Input: part model. Units: mm. Frame: model coordinates. A direction names the side the tool comes from. Give positions to 0.01 mm unless a question says otherwise; leave off trailing zeros. Loops run counter-clockwise (first coordinate to the right, second up) from the corner with the lowest first, then second, coordinate; pieces in that order, holes last. Notation, with made-up numbers: M 78,-28 L 82,-28 A21 cw 82,3 Z; hole C -21.5,55.25 d8. An arc over 180 degrees is marked long. One line per item, written item: value. Start each with the question number.
(1) Pin query (flat end, axial travel): P1, Ø4, axis at y = 87, z = -4, coming from the -X side; P2, Ø4, axis at y = 87.5, z = -4, coming from the -X side; P3, Ø3, axis at x = -11, z = -5, coming from the -Y side; P4, Ø10, axis at x = 0.5, y = 96, coming from the +Z side. Return the tip coordinate at first contact, or that it passes through.
(2) Section C-C on x = -9. Output: boundary loops of the cut face in (y, z).
(3) Section A-A on y = 94.5. Output: boundary loops of the cut face in (x, z).
(4) Pull-direction query (Y, two-part tool) for faces 1 (the flat face through (-9, 98.264, -5)), 2 (the cylindrical face through (-14.457, 98.836, -4.93)), 3 (the flat face through (2.38, 84.51, -4.93)); classes: released by +Y, released by -Y, zero draft, split by the parting line, or undercut.
(5) Section B-B on y = 92.25. Output: boundary loops of the cut face in (x, z), plus the area to 4 significant figures.
(6) Ray query, line 1 along X through (y, z) = (96.5, -1.25); line 2 along X through (y, z) = (85.5, -3.25); line 3 along Y through (x, z) = (-1, -6.75). Return the intervals inside material, ascending. Write a range as from..to.
(7) Access query for faces 4 (the flat face through (1.397, 86.815, -4.93)), 5 (the flat face through (-1.073, 83, -5)), 6 (the flat face through (-13.42, 87.23, -4.93)). Directions: +Z, -Z, +X, -X, +Y, -Y. A direction counts if a zero-diameter tool reaches every point of the face in a straight line with its end or side. Return the directions, or none.
```python
from build123d import *

# Parameters (mm, degrees)
BOSS_EXTRUDE1_DEPTH = 10


# Read off the part's stored shape, not the designer's step: Imported1
with BuildPart() as part:
    # Sketch5 → Boss-Extrude1 (new body)
    with BuildSketch(Plane.XY):
        with BuildLine():
            Line((-6.05700016, 98.805000305), (-6.127999783, 98.944999695))
            Line((-6.127999783, 98.944999695), (-6.152999878, 99.099998474))
            Line((-6.152999878, 99.099998474), (-6.127999783, 99.255996704))
            Line((-6.127999783, 99.255996704), (-6.123951545, 99.263979588))
            Line((-6.123951545, 99.263979588), (-13.408000231, 99.263979588))
            ThreePointArc((-13.408000231, 99.263979588), (-14.468660403, 98.82463976), (-14.908000231, 97.763979588))
            Line((-14.908000231, 97.763979588), (-14.908000231, 93.983181661))
            ThreePointArc((-14.908000231, 93.983181661), (-14.890789829, 93.756609361), (-14.839553555, 93.535236262))
            Line((-14.839553555, 93.535236262), (-13.37100029, 88.842002869))
            Line((-13.37100029, 88.842002869), (-13.322039604, 88.843772888))
            Line((-13.322039604, 88.843772888), (-13.524080276, 85.57485199))
            Line((-13.524080276, 85.57485199), (-13.550000191, 84.919998169))
            Line((-13.550000191, 84.919998169), (-13.409000397, 84.103996277))
            Line((-13.409000397, 84.103996277), (-12.994999886, 83.488998413))
            Line((-12.994999886, 83.488998413), (-12.32199955, 83.050003052))
            Line((-12.32199955, 83.050003052), (-11.402999878, 82.754997253))
            Line((-11.402999878, 82.754997253), (-10.253000259, 82.577003479))
            Line((-10.253000259, 82.577003479), (-10.078000069, 82.565231323))
            Line((-10.078000069, 82.565231323), (-10.078000069, 83.426826477))
            Line((-10.078000069, 83.426826477), (-10.673000336, 83.518997192))
            Line((-10.673000336, 83.518997192), (-11.477000237, 83.777000427))
            Line((-11.477000237, 83.777000427), (-12.065999985, 84.162002563))
            Line((-12.065999985, 84.162002563), (-12.428999901, 84.699996948))
            Line((-12.428999901, 84.699996948), (-12.552000046, 85.414001465))
            Line((-12.552000046, 85.414001465), (-12.44299984, 88.178001404))
            Line((-12.44299984, 88.178001404), (-13.908000231, 93.263979588))
            Line((-13.908000231, 93.263979588), (-13.908000231, 98.263979588))
            Line((-13.908000231, 98.263979588), (-4.410530424, 98.263979588))
            Line((-4.410530424, 98.263979588), (-3.957890034, 98.267951965))
            Line((-3.957890034, 98.267951965), (-3.944104194, 98.263979588))
            Line((-3.944104194, 98.263979588), (2.807999849, 98.263979588))
            Line((2.807999849, 98.263979588), (2.807999849, 93.263979588))
            Line((2.807999849, 93.263979588), (1.343000054, 88.178001404))
            Line((1.343000054, 88.178001404), (1.452999949, 85.414001465))
            Line((1.452999949, 85.414001465), (1.328999996, 84.699996948))
            Line((1.328999996, 84.699996948), (0.966000021, 84.162002563))
            Line((0.966000021, 84.162002563), (0.377000004, 83.777000427))
            Line((0.377000004, 83.777000427), (-0.426999986, 83.518997192))
            Line((-0.426999986, 83.518997192), (-1.072999954, 83.418922424))
            Line((-1.072999954, 83.418922424), (-1.072999954, 82.56186676))
            Line((-1.072999954, 82.56186676), (-0.84799999, 82.577003479))
            Line((-0.84799999, 82.577003479), (0.301999986, 82.754997253))
            Line((0.301999986, 82.754997253), (1.220999956, 83.050003052))
            Line((1.220999956, 83.050003052), (1.894000053, 83.488998413))
            Line((1.894000053, 83.488998413), (2.308000088, 84.103996277))
            Line((2.308000088, 84.103996277), (2.450000048, 84.919998169))
            Line((2.450000048, 84.919998169), (2.431600094, 85.381187439))
            Line((2.431600094, 85.381187439), (2.438999891, 85.382003784))
            Line((2.438999891, 85.382003784), (2.248559952, 88.639091492))
            Line((2.248559952, 88.639091492), (3.742796809, 93.540116743))
            ThreePointArc((3.742796809, 93.540116743), (3.791609542, 93.756422636), (3.807999849, 93.977561235))
            Line((3.807999849, 93.977561235), (3.807999849, 97.763979588))
            ThreePointArc((3.807999849, 97.763979588), (3.368660021, 98.82463976), (2.307999849, 99.263979588))
            Line((2.307999849, 99.263979588), (-5.176048197, 99.263979588))
            Line((-5.176048197, 99.263979588), (-5.171999931, 99.255996704))
            Line((-5.171999931, 99.255996704), (-5.147999763, 99.099998474))
            Line((-5.147999763, 99.099998474), (-5.171999931, 98.944999695))
            Line((-5.171999931, 98.944999695), (-5.243000031, 98.805000305))
            Line((-5.243000031, 98.805000305), (-5.355000019, 98.694000244))
            Line((-5.355000019, 98.694000244), (-5.494999886, 98.622001648))
            Line((-5.494999886, 98.622001648), (-5.650000095, 98.597999573))
            Line((-5.650000095, 98.597999573), (-5.804999828, 98.622001648))
            Line((-5.804999828, 98.622001648), (-5.945000172, 98.694000244))
            Line((-5.945000172, 98.694000244), (-6.05700016, 98.805000305))
        make_face()
    extrude(amount=-BOSS_EXTRUDE1_DEPTH)


solid = part.part
```
Output values:
1. P1: stops at x = -13.55
1. P2: stops at x = -13.58
1. P3: stops at y = 82.57
1. P4: stops at z = 0
2. outline: M 98.26,-10 L 99.26,-10 L 99.26,0 L 98.26,0 Z
3. outline: M -14.91,-10 L -13.91,-10 L -13.91,0 L -14.91,0 Z; M 2.81,-10 L 3.81,-10 L 3.81,0 L 2.81,0 Z
4. face 1: undercut
4. face 2: released by +Y
4. face 3: released by -Y
5. outline: M -14.44,-10 L -13.62,-10 L -13.62,0 L -14.44,0 Z; M 2.52,-10 L 3.35,-10 L 3.35,0 L 2.52,0 Z
5. area: 16.55 mm²
6. line 1: x = -14.91..-13.91, 2.81..3.81
6. line 2: x = -13.53..-12.55, 1.45..2.43
6. line 3: y = 82.57..83.43, 98.26..99.26
7. face 4: +Z, -Z
7. face 5: +Z, -Z, -Y
7. face 6: +Z, -Z, -X
